Here's how the part is built. I have some questions about the finished solid (model axes, mm). A direction names the side the tool comes from. Coordinates: 2 decimals unless noted, no trailing zeros. Write each loop counter-clockwise with the first axis right and the second up, starting at its lowest first coordinate (ties: lowest second). Pieces come first, ordered by that corner, then holes. Notation, with made-up numbers: (14, 16) -> (20, 16) arc R19 cw to (20, 46) -> close; hole circle Ø1 at (8.25, -21.75). An arc over 180 degrees is marked (long way). Put each result on its own line as item: value.
```python
from build123d import *

# Parameters (mm, degrees)
SKETCH1_W            = 60
SKETCH1_H            = 30
SKETCH1_R            = 4
BOSS_EXTRUDE1_DEPTH  = 2.5
FILLET1_R            = 8
SKETCH3_R            = 4
BOSS_EXTRUDE2_DEPTH  = 9
SKETCH4_R            = 14
CUT_EXTRUDE1_DEPTH   = 4.5
FILLET2_R            = 2
FILLET2_OF_MIRROR1_R = 2


with BuildPart() as part:
    # Sketch1 → Boss-Extrude1 (new, symmetric)
    with BuildSketch(Plane.XY):
        Rectangle(SKETCH1_W, SKETCH1_H)
        with Locations((-20, 0)):
            Circle(SKETCH1_R, mode=Mode.SUBTRACT)
        with Locations(Location((20, 0, 0), (0, 0, 180))):
            Circle(SKETCH1_R, mode=Mode.SUBTRACT)
    extrude(amount=BOSS_EXTRUDE1_DEPTH, both=True)

    # Fillet1
    fillet1_edges = [part.edges().sort_by_distance(p)[0] for p in [
        (30, -15, 0),
        (-30, -15, 0),
        (-30, 15, 0),
        (30, 15, 0),
    ]]
    fillet(fillet1_edges, radius=FILLET1_R)

    # Sketch3 → Boss-Extrude2 (add, symmetric)
    with BuildSketch(Plane(origin=(0, 0, 0), x_dir=(0, 0, -1), z_dir=(1, 0, 0))):
        with BuildLine():
            Line((-2.5, 15), (-45.735238064, 3.415152876))
            ThreePointArc((-45.735238064, 3.415152876), (-54.574072829, -11.894158016), (-39.264761936, -20.732992781))
            Line((-39.264761936, -20.732992781), (-17.868941598, -15))
            Line((-17.868941598, -15), (-2.5, -15))
            Line((-2.5, -15), (-2.5, 15))
        make_face()
        with Locations((-42.5, -8.658919952)):
            Circle(SKETCH3_R, mode=Mode.SUBTRACT)
    extrude(amount=BOSS_EXTRUDE2_DEPTH, both=True)

    # Sketch4 → Cut-Extrude1 (cut)
    with BuildSketch(Plane(origin=(9, 0, 0), x_dir=(0, 0, -1), z_dir=(1, 0, 0))):
        with Locations((-42.5, -8.658919952)):
            Circle(SKETCH4_R)
    cut_extrude1 = extrude(amount=-CUT_EXTRUDE1_DEPTH, mode=Mode.SUBTRACT)

    # Fillet2
    fillet2_edges = [part.edges().sort_by_distance(p)[0] for p in [
        (6.75, -19.101200791, 33.174831321),
        (6.75, 5.046944867, 39.645307448),
    ]]
    fillet(fillet2_edges, radius=FILLET2_R)

    # Mirror1: Cut-Extrude1 across plane
    add(cut_extrude1.mirror(Plane(origin=(0, 0, 0), x_dir=(0, 0, 1), z_dir=(1, 0, 0))), mode=Mode.SUBTRACT)

    # Fillet2 of Mirror1
    fillet2_of_mirror1_edges = [part.edges().sort_by_distance(p)[0] for p in [
        (-6.75, -19.101200791, 33.174831321),
        (-6.75, 5.046944867, 39.645307448),
    ]]
    fillet(fillet2_of_mirror1_edges, radius=FILLET2_OF_MIRROR1_R)


solid = part.part
```
Item 1: Imagine slicing it at C-C on z = 42.5. Write out the boundary of the cut face in (x, y), then the cut area to 3 significant figures.
Output:
outline: (-4.5, -21.16) -> (4.5, -21.16) -> (4.5, -12.66) -> (-4.5, -12.66) -> close; (-4.5, -4.66) -> (4.5, -4.66) -> (4.5, 4.28) -> (-4.5, 4.28) -> close
area: 157 mm²
Item 2: If we mould it in two halves opening along Z, with no side actions, what happens to faces 1 (the flat face through (0, 0, -2.5)), 2 (the cylindrical face through (-0.06, -5.96, 45.45)), 3 (the cylindrical face through (6.78, -5.17, 28.94))? For each: released by +Z, released by -Z, zero draft, split by the parting line, or undercut.
Output:
face 1: released by -Z
face 2: undercut
face 3: released by +Z
Item 3: Imagine slicing it at A-A on x = 20. Write out the boundary of the cut face in (y, z).
Output:
outline: (-15, -2.5) -> (-4, -2.5) -> (-4, 2.5) -> (-15, 2.5) -> close; (4, -2.5) -> (15, -2.5) -> (15, 2.5) -> (4, 2.5) -> close
Item 4: Imagine slicing it at B-B on y = 0. Write out the boundary of the cut face in (x, z), then the cut area to 3 significant figures.
Output:
outline: (-30, -2.5) -> (-24, -2.5) -> (-24, 2.5) -> (-30, 2.5) -> close; (-16, -2.5) -> (16, -2.5) -> (16, 2.5) -> (9, 2.5) -> (9, 31.5) -> (4.5, 31.5) -> (4.5, 51.52) -> (-4.5, 51.52) -> (-4.5, 31.5) -> (-9, 31.5) -> (-9, 2.5) -> (-16, 2.5) -> close; (24, -2.5) -> (30, -2.5) -> (30, 2.5) -> (24, 2.5) -> close
area: 922 mm²
Item 5: Imagine slicing it at D-D on x = 8. Write out the boundary of the cut face in (y, z).
Output:
outline: (-17.61, 27.6) -> (-15, 17.87) -> (-15, -2.5) -> (15, -2.5) -> (15, 2.5) -> (6.54, 34.07) arc R2 ccw to (2.95, 34.67) arc R14 cw to (-14.8, 29.92) arc R2 ccw to start
Item 6: Please list where these lines run through material, in increasing order: line 1 along Y through (x, z) = (-20, 0); line 2 along Z through (x, y) = (12.5, 3); line 3 along X through (y, z) = (-7.5, 24). Write a range as from..to.
Output:
line 1: y = -15..-4, 4..15
line 2: z = -2.5..2.5
line 3: x = -9..9
Item 7: Which directions (+Z, -Z, +X, -X, +Y, -Y) give clear straight access to the entire face, cutting with the end or side of a thin tool? Please do faces 4 (the flat face through (30, 0, 0)), 5 (the cylindrical face through (-6.781, 4.969, 35.523)), 6 (the cylindrical face through (-27.719, 12.594, -0.035)), 7 (the cylindrical face through (6.781, 4.906, 35.534)), 8 (the flat face through (9, -1, 16)).
Output:
face 4: +Z, -Z, +X, +Y, -Y
face 5: +Z, -X
face 6: +Z, -Z, -X, +Y
face 7: +Z, +X
face 8: +Z, +X, +Y, -Y
Item 8: For P1, Ø5, axis at y = -11, z = 44.5, coming from the -X side; P2, Ø2, axis at y = -14, z = 9, coming from the +X side; P3, Ø13.5, axis at y = -13.5, z = 35.5, coming from the -X side; P4, Ø7, axis at x = -20, y = 0, coming from the +Z side, each with a flat end and sliding along its axis, tell me the tip position at first contact or that it passes through.
Output:
P1: stops at x = -4.5
P2: stops at x = 9
P3: stops at x = -9
P4: passes through
